```python
from build123d import *

# Parameters (mm, degrees)
SKETCH_1_W          = 51
SKETCH_1_H          = 41
SKETCH_1_R          = 1.25
EXTRUDE_1_DEPTH     = 3.4
SKETCH_2_R          = 1
EXTRUDE_2_DEPTH     = 2.5
SKETCH_3_W          = 14.5
SKETCH_3_H          = 35.737354226
CUT_EXTRUDE_1_DEPTH = 1.4
EXTRUDE_4_DEPTH     = 2
FILLET_1_R          = 8
FILLET_2_R          = 4
SKETCH_6_R          = 2
CUT_EXTRUDE_2_DEPTH = 1.2
CUT_EXTRUDE_3_DEPTH = 4
FILLET_3_R          = 3
SKETCH_9_R          = 2
CUT_EXTRUDE_4_DEPTH = 0.8
SKETCH_10_R         = 2.5
CUT_EXTRUDE_5_DEPTH = 1.4
CHAMFER_1_SIZE      = 0.8
FILLET_4_R          = 4
FILLET_5_R          = 5
CUT_EXTRUDE_6_DEPTH = 10
FILLET_6_R          = 1


with BuildPart() as part:
    # 草图1 → 凸台-拉伸1 (new body)
    with BuildSketch(Plane(origin=(0, 0, 0), x_dir=(1, 0, 0), z_dir=(0, 1, 0))):
        Rectangle(SKETCH_1_W, SKETCH_1_H)
        with Locations(Location((-22.5, 6, 0), (0, 0, 270))):
            Circle(SKETCH_1_R, mode=Mode.SUBTRACT)
        with Locations(Location((-22.5, -6, 0), (0, 0, 90))):
            Circle(SKETCH_1_R, mode=Mode.SUBTRACT)
        with Locations(Location((-6.5, 6, 0), (0, 0, 270))):
            Circle(SKETCH_1_R, mode=Mode.SUBTRACT)
        with Locations(Location((-6.5, -6, 0), (0, 0, 90))):
            Circle(SKETCH_1_R, mode=Mode.SUBTRACT)
    extrude(amount=EXTRUDE_1_DEPTH)

    # 草图2 → 凸台-拉伸2 (add)
    with BuildSketch(Plane(origin=(25.5, 0, 0), x_dir=(0, 0, -1), z_dir=(1, 0, 0))):
        with BuildLine():
            Line((-20.5, 0), (20.5, 0))
            Line((20.5, 0), (20.5, -100))
            Line((20.5, -100), (9.43808773, -100))
            ThreePointArc((9.43808773, -100), (0, -94.65), (-9.43808773, -100))
            Line((-9.43808773, -100), (-20.5, -100))
            Line((-20.5, -100), (-20.5, 0))
        make_face()
        with Locations((-10.25, -97.35)):
            Circle(SKETCH_2_R, mode=Mode.SUBTRACT)
        with Locations(Location((10.25, -97.35, 0), (0, 0, 180))):
            Circle(SKETCH_2_R, mode=Mode.SUBTRACT)
        with Locations((10.25, -76.65)):
            Circle(SKETCH_2_R, mode=Mode.SUBTRACT)
        with Locations(Location((-10.25, -76.65, 0), (0, 0, 180))):
            Circle(SKETCH_2_R, mode=Mode.SUBTRACT)
    extrude(amount=-EXTRUDE_2_DEPTH)

    # 草图3 → 切除-拉伸1 (cut)
    with BuildSketch(Plane(origin=(25.5, 0, 0), x_dir=(0, 0, -1), z_dir=(1, 0, 0))):
        with Locations((0, -88.518677113)):
            Rectangle(SKETCH_3_W, SKETCH_3_H)
    extrude(amount=-CUT_EXTRUDE_1_DEPTH, mode=Mode.SUBTRACT)

    # 草图5 → 凸台-拉伸4 (add)
    with BuildSketch(Plane(origin=(0, 0, -20.5), x_dir=(-1, 0, 0), z_dir=(0, 0, -1))):
        with BuildLine():
            Line((-25.5, 3.4), (19.5, 3.4))
            Line((19.5, 3.4), (19.5, 0))
            add(Edge.make_bspline(
                [(19.5, 0), (10.67122189, -5.3692624), (2.779429236, -18.193392293), (-14.23746955, -82.475470635), (-23, -82.805044976)],
                knots=[0, 0, 0, 0.396049025, 0.788579615, 1, 1, 1], degree=2))
            Line((-23, -82.805044976), (-25.5, -82.805044976))
            Line((-25.5, -82.805044976), (-25.5, 3.4))
        make_face()
    extrude_4 = extrude(amount=-EXTRUDE_4_DEPTH)

    # 镜向3: 凸台-拉伸4 across plane
    add(extrude_4.mirror(Plane.XY))

    # 圆角1
    fillet_1_edges = [part.edges().sort_by_distance(p)[0] for p in [
        (-25.5, 1.7, -20.5),
        (-25.5, 1.7, 20.5),
    ]]
    fillet(fillet_1_edges, radius=FILLET_1_R)

    # 圆角2
    fillet_2_edges = [part.edges().sort_by_distance(p)[0] for p in [
        (25.5, 3.4, 0),
        (23, 0, 0),
    ]]
    fillet(fillet_2_edges, radius=FILLET_2_R)

    # 草图6 → 切除-拉伸2 (cut)
    with BuildSketch(Plane.ZY.offset(-23)):
        with Locations((10.25, -97.35)):
            Circle(SKETCH_6_R)
        with Locations((-10.25, -97.35)):
            Circle(SKETCH_6_R)
    extrude(amount=-CUT_EXTRUDE_2_DEPTH, mode=Mode.SUBTRACT)

    # 草图8 → 切除-拉伸3 (cut)
    with BuildSketch(Plane(origin=(25.5, 0, 0), x_dir=(0, 0, -1), z_dir=(1, 0, 0))):
        Polygon((14, -102.818047241), (14, -92), (23.468492482, -92), (23.468492482, -110.008191191), (-23.468492482, -110.008191191), (-23.468492482, -92), (-14, -92), (-14, -102.818047241), align=None)
    extrude(amount=-CUT_EXTRUDE_3_DEPTH, mode=Mode.SUBTRACT)

    # 圆角3
    fillet_3_edges = [part.edges().sort_by_distance(p)[0] for p in [
        (24.25, -100, 14),
        (24.25, -100, -14),
        (24.25, -92, -14),
        (24.25, -92, 14),
    ]]
    fillet(fillet_3_edges, radius=FILLET_3_R)

    # 草图9 → 切除-拉伸4 (cut)
    with BuildSketch(Plane.ZY.offset(-23)):
        with Locations((10.25, -76.65)):
            Circle(SKETCH_9_R)
        with Locations(Location((-10.25, -76.65, 0), (0, 0, 180))):
            Circle(SKETCH_9_R)
    extrude(amount=-CUT_EXTRUDE_4_DEPTH, mode=Mode.SUBTRACT)

    # 草图10 → 切除-拉伸5 (cut)
    with BuildSketch(Plane(origin=(0, 0, 0), x_dir=(-1, 0, 0), z_dir=(0, -1, 0))):
        with Locations(Location((6.5, -6, 0), (0, 0, 90))):
            Circle(SKETCH_10_R)
        with Locations(Location((22.5, -6, 0), (0, 0, 270))):
            Circle(SKETCH_10_R)
        with Locations(Location((6.5, 6, 0), (0, 0, 270))):
            Circle(SKETCH_10_R)
        with Locations(Location((22.5, 6, 0), (0, 0, 90))):
            Circle(SKETCH_10_R)
    extrude(amount=-CUT_EXTRUDE_5_DEPTH, mode=Mode.SUBTRACT)

    # 倒角1
    chamfer_1_edges = [part.edges().sort_by_distance(p)[0] for p in [
        (24.25, -92, 20.5),
        (24.25, -92, -20.5),
    ]]
    chamfer(chamfer_1_edges, length=CHAMFER_1_SIZE)

    # 圆角4
    fillet_4_edges = [part.edges().sort_by_distance(p)[0] for p in [
        (-0.25, 0, -18.5),
        (21.828427125, -1.171572875, -18.5),
        (-0.25, 0, 18.5),
        (21.828427125, -1.171572875, 18.5),
        (23, -43.402522488, -18.5),
        (23, -43.402522488, 18.5),
    ]]
    fillet(fillet_4_edges, radius=FILLET_4_R)

    # 圆角5
    fillet_5_edges = [part.edges().sort_by_distance(p)[0] for p in [
        (23, -82.805044976, 16.5),
        (23, -82.805044976, -16.5),
        (-19.5, 0, 16.5),
        (-19.5, 0, -16.5),
    ]]
    fillet(fillet_5_edges, radius=FILLET_5_R)

    # 草图12 → 切除-拉伸6 (cut)
    with BuildSketch(Plane.ZY.offset(-23)):
        with BuildLine():
            Line((-6.873863542, -11), (-9, -11))
            Line((-9, -11), (-9, -21))
            Line((-9, -21), (-6.873863542, -21))
            ThreePointArc((-6.873863542, -21), (0, -24.5), (6.873863542, -21))
            Line((6.873863542, -21), (9, -21))
            Line((9, -21), (9, -11))
            Line((9, -11), (6.873863542, -11))
            ThreePointArc((6.873863542, -11), (0, -7.5), (-6.873863542, -11))
        make_face()
    extrude(amount=-CUT_EXTRUDE_6_DEPTH, mode=Mode.SUBTRACT)

    # 圆角6
    fillet_6_edges = [part.edges().sort_by_distance(p)[0] for p in [
        (24.25, -21, -9),
        (24.25, -11, -9),
        (24.25, -11, -6.873863542),
        (24.25, -11, 6.873863542),
        (24.25, -11, 9),
        (24.25, -21, 9),
        (24.25, -21, 6.873863542),
        (24.25, -21, -6.873863542),
    ]]
    fillet(fillet_6_edges, radius=FILLET_6_R)


solid = part.part
```
Could you check a few things on this model? Use its own coordinates, in mm. A direction names the side the tool comes from. Coordinates: 2 decimals unless noted, no trailing zeros. Loops run counter-clockwise (first coordinate to the right, second up) from the corner with the lowest first, then second, coordinate; pieces in that order, holes last.
1) Which directions (+Z, -Z, +X, -X, +Y, -Y) give clear straight access to the entire face, cutting with the end or side of a thin tool? Please do faces 1 (the face through (24, -96, 14)), 2 (the face through (24, -16, 9)), 3 (the face through (-5, 1.4, 5)).
Reported:
face 1: +Z, +X, -X, -Y
face 2: +X, -X
face 3: -Y
2) Thinking about a two-plate mould opening in Y: for faces 4 (the face through (10, -34, 18.5)), 5 (the face through (23.71, -94.65, -0.16)), 6 (the face through (24, -16, -9)), which applies, released by +Y, released by -Y, zero draft, split by the parting line, or undercut?
Reported:
face 4: zero draft
face 5: released by -Y
face 6: undercut
3) Imagine slicing it at A-A (x = -22.5). List the corners of the cut face in (y, z) for me (3 decimals), and give its area (3 significant figures).
Reported:
outline: (0, -18.745) - (3.4, -18.745) - (3.4, -7.25) - (1.4, -7.25) - (1.4, -8.5) - (0, -8.5) - close; (0, -3.5) - (1.4, -3.5) - (1.4, -4.75) - (3.4, -4.75) - (3.4, 4.75) - (1.4, 4.75) - (1.4, 3.5) - (0, 3.5) - close; (0, 8.5) - (1.4, 8.5) - (1.4, 7.25) - (3.4, 7.25) - (3.4, 18.745) - (0, 18.745) - close
area: 103 mm2
4) Please list where these lines run through material, in increasing order: line 1 along Z through (x, y) = (24.25, -76.65); line 2 along Y through (x, z) = (24, -10); line 3 along Z through (x, y) = (16, -5.5).
Reported:
line 1: z = -20.5 to -11.25, -9.25 to -7.25, 7.25 to 9.25, 11.25 to 20.5
line 2: y = -100 to -99.33, -95.37 to -77.62, -75.68 to 2.52
line 3: z = -20.5 to -18.5, 18.5 to 20.5
5) Will these pins go through, and if not, where does the flat tip stop? pin 1 Ø1.5 at (x, z) = (24.5, 1.5) entering from -Y; pin 2 Ø12.5 at (y, z) = (-73, -3) entering from -X; pin 3 Ø1 at (x, y) = (25, -96) entering from +Z; pin 4 Ø12 at (x, y) = (3, -75.5) entering from +Z.
Reported:
pin 1: stops at y = -94.86
pin 2: stops at x = 23
pin 3: stops at z = 14
pin 4: passes through
6) Imagine slicing it at B-B (y = -76.65). State how many separate pieces and enclosed holes the cut face has, and give its area (3 significant figures).
Reported:
separate pieces: 3
enclosed holes: 0
area: 109 mm2
